```python
from build123d import *

# Parameters (mm, degrees)
BOX037_W               = 100
BOX037_H               = 2
BOX037_DEPTH           = 60
CYLINDER090_R          = 28
CYLINDER090_DEPTH      = 28
BOX035_W               = 40
BOX035_H               = 20.2
BOX035_DEPTH           = 10
BOX035_PLACEMENT_ANGLE = 45
BOX036_W               = 34
BOX036_H               = 22
BOX036_DEPTH           = 10
BOX036_PLACEMENT_ANGLE = 45
BOX033_W               = 26.5
BOX033_H               = 20.2
BOX033_DEPTH           = 28
BOX033_PLACEMENT_ANGLE = 45
BOX034_W               = 31.5
BOX034_H               = 28
BOX034_DEPTH           = 28
BOX034_PLACEMENT_ANGLE = 45


with BuildPart() as face006:
    # Box037 → Box037 (new body)
    with BuildSketch(Plane(origin=(-33, 47.5, -59), x_dir=(1, 0, 0), z_dir=(0, 0, 1))):
        with Locations((50, 1)):
            Rectangle(BOX037_W, BOX037_H)
    extrude(amount=BOX037_DEPTH)


with BuildPart() as cylinder090:
    # Cylinder090 → Cylinder090 (new body)
    with BuildSketch(Plane.XY.offset(-28)):
        Circle(CYLINDER090_R)
    extrude(amount=CYLINDER090_DEPTH)


with BuildPart() as cube017:
    # Box035 → Box035 (new body)
    with BuildSketch(Plane.XY):
        with Locations((20, 10.1)):
            Rectangle(BOX035_W, BOX035_H)
    extrude(amount=BOX035_DEPTH)


with BuildPart() as cube017_1:
    # Box035 placement: moved
    add(cube017.part.moved(Location((20, 5.8, -10))).rotate(Axis((20, 5.8, -10), (0, 0, 1)), BOX035_PLACEMENT_ANGLE))


with BuildPart() as servo_secure002:
    # Box036 → Box036 (new body)
    with BuildSketch(Plane.XY):
        with Locations((17, 11)):
            Rectangle(BOX036_W, BOX036_H)
    extrude(amount=BOX036_DEPTH)


with BuildPart() as servo_secure002_1:
    # Box036 placement: moved
    add(servo_secure002.part.moved(Location((23, 7.5, -10))).rotate(Axis((23, 7.5, -10), (0, 0, 1)), BOX036_PLACEMENT_ANGLE))

    # Cut092: cut Cube017
    add(cube017_1.part, mode=Mode.SUBTRACT)


with BuildPart() as inner:
    # Box033 → Box033 (new body)
    with BuildSketch(Plane.XY):
        with Locations((13.25, 10.1)):
            Rectangle(BOX033_W, BOX033_H)
    extrude(amount=BOX033_DEPTH)


with BuildPart() as inner_1:
    # Box033 placement: moved
    add(inner.part.moved(Location((24.2, 10, -28))).rotate(Axis((24.2, 10, -28), (0, 0, 1)), BOX033_PLACEMENT_ANGLE))


with BuildPart() as cut095:
    # Box034 → Box034 (new body)
    with BuildSketch(Plane.XY):
        with Locations((15.75, 14)):
            Rectangle(BOX034_W, BOX034_H)
    extrude(amount=BOX034_DEPTH)


with BuildPart() as cut095_1:
    # Box034 placement: moved
    add(cut095.part.moved(Location((27.2, 7, -28))).rotate(Axis((27.2, 7, -28), (0, 0, 1)), BOX034_PLACEMENT_ANGLE))

    # Cut091: cut inner
    add(inner_1.part, mode=Mode.SUBTRACT)

    # Cut093: cut servo-secure002
    add(servo_secure002_1.part, mode=Mode.SUBTRACT)

    # Cut094: cut Cylinder090
    add(cylinder090.part, mode=Mode.SUBTRACT)

    # Cut095: cut face006
    add(face006.part, mode=Mode.SUBTRACT)


solid = cut095_1.part
```
Design review of the part built by this model. Coordinates are the model's own, in mm. A direction names the side the tool comes from. Give positions to 0.01 mm unless a question says otherwise; leave off trailing zeros. Order: outer loops, then holes, each group sorted by start corner. A loop starts at its lowest first (then second) coordinate and runs counter-clockwise, first axis right, second up. Notation, with made-up numbers: M 56.25,9 L 70.25,9 A25 ccw 70.25,47 Z; hole C 20,23 d3. An arc over 180 degrees is marked long. One line per question, with ' | ' between items. Start each with the question number.
Q1. For pin 1 Ø2 at (y, z) = (19, -8) entering from -X; pin 2 Ø6 at (x, z) = (36, -11) entering from +Y; pin 3 Ø5 at (x, z) = (17, -12.5) entering from -Y, all flat-tipped, find the tip position at first contact; note any pin that passes through.
Q2. We need section A-A (x = 26.5). Write out the cut boundary in (y, z), plus the area to 3 significant figures.
Q3. We need section C-C (y = 38.5). Write out the cut boundary in (x, z), plus the area to 3 significant figures.
Q4. For L1, parallel to X at y = 35.5, z = -20.75; L2, parallel to X at y = 36, z = -12; L3, parallel to Y at x = 41, z = -12, list the stretches that pass through material, from the lowest coordinate up. Write a range as [from, to].
Q5. We need section B-B (z = -2). Write out the cut boundary in (x, y), plus the area to 3 significant figures.
Q6. We need section D-D (y = 45). Write out the cut boundary in (x, z).
Q7. Machinability: for faces 1 (the face through (30, 47.5, -14)), 2 (the face through (19.839, 34.206, -19.126)), 3 (the face through (21, 36, -10)), which of the approach directions +Z, -Z, +X, -X, +Y, -Y give a long, thin tool a straight path to every point of the face, cutting with its end or side? Answer none if there is none.
Returned:
1) pin 1: x = 33.5 | pin 2: y = 45.75 | pin 3: y = 28.87
2) outline: M 9.04,-28 L 12.3,-28 L 12.3,-10 L 11,-10 L 11,0 L 9.04,0 Z; M 40.87,-28 L 45.9,-28 L 45.9,0 L 42.11,0 L 42.11,-10 L 40.87,-10 Z | area: 207 mm2
3) outline: M 19.1,-28 L 24.13,-28 L 24.13,-10 L 22.89,-10 L 22.89,0 L 19.1,0 Z; M 33.18,-28 L 40.25,-28 L 40.25,0 L 33.18,0 Z | area: 326 mm2
4) L1: [16.1, 21.13], [36.18, 43.25] | L2: [16.6, 21.63], [35.68, 42.75] | L3: [20.8, 26.8], [30.68, 37.75]
5) outline: M 7.56,26.96 A28 cw 10.39,26 L 31.49,47.1 L 32.11,46.48 L 28.65,43.02 L 42.94,28.74 L 46.39,32.19 L 47.04,31.54 L 25.97,10.47 A28 cw 27.08,7.12 L 27.2,7 L 49.47,29.27 L 31.25,47.5 L 28.1,47.5 Z | area: 283 mm2
6) outline: M 25.6,-28 L 33.75,-28 L 33.75,0 L 30.63,0 L 30.63,-10 L 29.39,-10 L 29.39,0 L 25.6,0 Z
7) face 1: +Z, -Z, +X, -X, +Y | face 2: +Z, -Z | face 3: +Z
